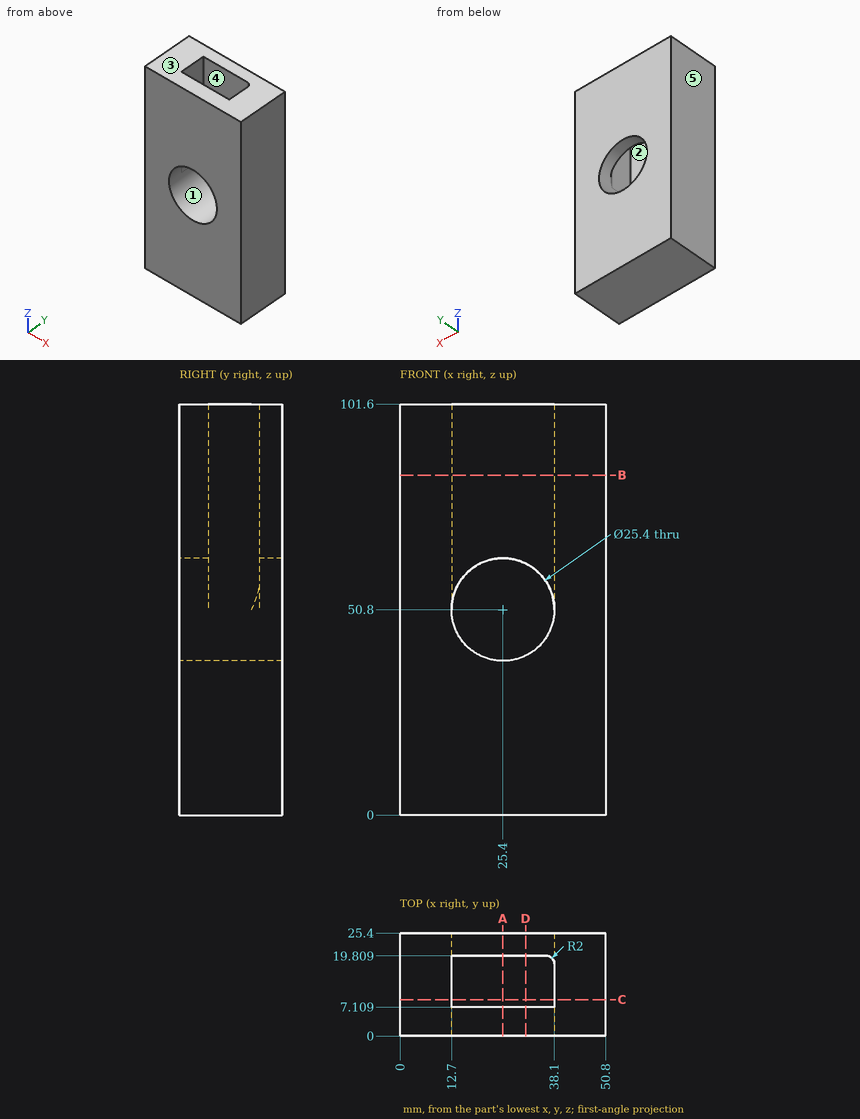
For this review, use the dimensioned drawing (mm, ordinates from the lowest corner) and the shaded views. A direction names the side the tool comes from. Round coordinates to 2 decimals unless told otherwise and drop trailing zeros. Write each loop counter-clockwise with the first axis right and the second up, starting at its lowest first coordinate (ties: lowest second). Pieces come first, ordered by that corner, then holes. Notation, with made-up numbers: (20, -25) - (62, -25) arc R28 cw to (62, 12) - close; hole circle Ø1 at (25, 73). An arc over 180 degrees is marked (long way). One line per item, written item: value. Start each with the question number.
1. The part is to be moulded in two halves that separate along Z. For the marked faces 1, 2 and 3, say which applies: released by +Z, released by -Z, zero draft, split by the parting line, or undercut.
2. To check wall thickness, follow L1, parallel to X at y = 18, z = 50.8; L2, parallel to Y at x = 33, z = 82; L3, parallel to Z at x = 25.4, y = 20. State the ranges of each line that lie inside material, in increasing order. Write a range as from..to.
3. Consider section B-B on z = 84. Write out the cut boundary in (x, y).
4. Consider section C-C on y = 9. Write out the cut boundary in (x, z).
5. Clearance check with flat-ended pins moving along their axes: P1, Ø1.5, axis at y = 20.5, z = 64.5, coming from the -X side; P2, Ø1, axis at x = 31.5, y = 10, coming from the +Z side. State where each tip first meets the part, or that it passes through.
6. Machinability: for the marked faces 4 and 5, which of the approach directions +Z, -Z, +X, -X, +Y, -Y give a long, thin tool a straight path to every point of the face, cutting with its end or side? Answer none if there is none.
7. Consider section A-A on x = 25.4. Write out the cut boundary in (y, z), and give its area (3 significant figures).
8. Consider section D-D on x = 31. Write out the cut boundary in (y, z).
Checks:
1. face 1: undercut
1. face 2: zero draft
1. face 3: released by +Z
2. L1: x = 0..12.7, 38.1..50.8
2. L2: y = 0..7.11, 19.81..25.4
2. L3: z = 0..38.1, 63.5..101.6
3. outline: (0, 0) - (50.8, 0) - (50.8, 25.4) - (0, 25.4) - close; hole (12.7, 7.11) - (38.1, 7.11) - (38.1, 17.81) arc R2 ccw to (36.1, 19.81) - (12.7, 19.81) - close
4. outline: (0, 0) - (50.8, 0) - (50.8, 101.6) - (38.1, 101.6) - (38.1, 50.8) arc R12.7 cw to (12.7, 50.8) - (12.7, 101.6) - (0, 101.6) - close
5. P1: stops at x = 0
5. P2: stops at z = 39.95
6. face 4: +Z
6. face 5: +Z, -Z, -X, +Y, -Y
7. outline: (0, 0) - (25.4, 0) - (25.4, 38.1) - (0, 38.1) - close; (0, 63.5) - (7.11, 63.5) - (7.11, 101.6) - (0, 101.6) - close; (19.81, 63.5) - (25.4, 63.5) - (25.4, 101.6) - (19.81, 101.6) - close
7. area: 1,450 mm^2
8. outline: (0, 0) - (25.4, 0) - (25.4, 39.4) - (0, 39.4) - close; (0, 62.2) - (7.11, 62.2) - (7.11, 101.6) - (0, 101.6) - close; (19.81, 62.2) - (25.4, 62.2) - (25.4, 101.6) - (19.81, 101.6) - close
